```python
from build123d import *

# Parameters (mm, degrees)
SKETCH1_R           = 3.25
BOSS_EXTRUDE1_DEPTH = 12.5
SKETCH2_R           = 1.75
CUT_EXTRUDE1_DEPTH  = 2.5
SKETCH6_R           = 4.8
BOSS_EXTRUDE2_DEPTH = 5
FILLET1_R           = 0.75


with BuildPart() as part:
    # Sketch1 → Boss-Extrude1 (new body)
    with BuildSketch(Plane(origin=(0, 0, 0), x_dir=(1, 0, 0), z_dir=(0, 1, 0))):
        Circle(SKETCH1_R)
    extrude(amount=BOSS_EXTRUDE1_DEPTH)

    # Sketch2 → Cut-Extrude1 (cut)
    with BuildSketch(Plane.XZ):
        Circle(SKETCH2_R)
    extrude(amount=-CUT_EXTRUDE1_DEPTH, mode=Mode.SUBTRACT)

    # Sketch6 → Boss-Extrude2 (add)
    with BuildSketch(Plane(origin=(0, 12.5, 0), x_dir=(1, 0, 0), z_dir=(0, 1, 0))):
        Circle(SKETCH6_R)
    extrude(amount=BOSS_EXTRUDE2_DEPTH)

    # Fillet1
    fillet1_edges = [part.edges().sort_by_distance(p)[0] for p in [
        (-4.8, 17.5, 0),
    ]]
    fillet(fillet1_edges, radius=FILLET1_R)


solid = part.part
```
Here's how the part is built. I have some questions about the finished solid (model axes, mm). A direction names the side the tool comes from. Round coordinates to 2 decimals unless told otherwise and drop trailing zeros. Order: outer loops, then holes, each group sorted by start corner. A loop starts at its lowest first (then second) coordinate and runs counter-clockwise, first axis right, second up. Notation, with made-up numbers: (-8.5, 41) -> (14.5, 41) arc R21 ccw to (14.5, 51) -> close; hole circle Ø5 at (72.25, 49). An arc over 180 degrees is marked (long way). Use a Markdown table: item, result. Add a question column.
(1) Suppose I cut it at C-C, the plane y = 5. Please give me the cut outline in (x, z).
(2) Suppose I cut it at D-D, the plane y = 12.75. Please give me the cut outline in (x, z), and give its area (3 significant figures).
(3) Suppose I cut it at A-A, the plane x = 0. Please give me the cut outline in (y, z), and give its area (3 significant figures).
(4) For faces 1 (the face through (1.4, 0, 1.4)), 2 (the face through (-2.579, 6.162, 1.978)), which set-ups out of +Z, -Z, +X, -X, +Y, -Y let a thin tool reach every point of the face, with its end or its side?
(5) I need wall thicknesses on line 1 along Z through (x, y) = (0, 0.95); line 2 along Y through (x, z) = (0.5, 3.75); line 3 along Z through (x, y) = (0, 8). Which ranges of each line are inside material? Lowest first, please.
(6) For pin 1 Ø1.5 at (x, y) = (-2.5, 12.5) entering from +Z; pin 2 Ø1 at (x, z) = (-3.5, 3) entering from -Y; pin 3 Ø3 at (x, z) = (0, 0) entering from -Y, each with a flat end and sliding along its axis, tell me the tip position at first contact or that it passes through.
(7) Suppose I cut it at B-B, the plane z = 0. Please give me the cut outline in (x, y), and give its area (3 significant figures).
(8) If we mould it in two halves opening along Z, with no side actions, what happens to faces 3 (the face through (2.58, 14.6, -4.05)), 4 (the face through (0, 2.5, 0)), 5 (the face through (0, 17.5, 0))? For each: released by +Z, released by -Z, zero draft, split by the parting line, or undercut.
Verdict:
| question | item | result |
|---|---|---|
| 1 | outline | circle Ø6.5 at (0, 0) |
| 2 | outline | circle Ø9.6 at (0, 0) |
| 2 | area | 72.4 mm2 |
| 3 | outline | (0, -3.25) -> (12.5, -3.25) -> (12.5, -4.8) -> (16.75, -4.8) arc R0.75 ccw to (17.5, -4.05) -> (17.5, 4.05) arc R0.75 ccw to (16.75, 4.8) -> (12.5, 4.8) -> (12.5, 3.25) -> (0, 3.25) -> (0, 1.75) -> (2.5, 1.75) -> (2.5, -1.75) -> (0, -1.75) -> close |
| 3 | area | 120 mm2 |
| 4 | face 1 | +Z, -Z, +X, -X, -Y |
| 4 | face 2 | -Y |
| 5 | line 1 | -3.25 to -1.75, 1.75 to 3.25 |
| 5 | line 2 | 12.5 to 17.5 |
| 5 | line 3 | -3.25 to 3.25 |
| 6 | pin 1 | z = 4.47 |
| 6 | pin 2 | y = 12.5 |
| 6 | pin 3 | y = 2.5 |
| 7 | outline | (-4.8, 12.5) -> (-3.25, 12.5) -> (-3.25, 0) -> (-1.75, 0) -> (-1.75, 2.5) -> (1.75, 2.5) -> (1.75, 0) -> (3.25, 0) -> (3.25, 12.5) -> (4.8, 12.5) -> (4.8, 16.75) arc R0.75 ccw to (4.05, 17.5) -> (-4.05, 17.5) arc R0.75 ccw to (-4.8, 16.75) -> close |
| 7 | area | 120 mm2 |
| 8 | face 3 | split by the parting line |
| 8 | face 4 | undercut |
| 8 | face 5 | zero draft |
